from build123d import *

# Parameters (mm, degrees)
F2_R     = 6.35
F3_DEPTH = 6.732


with BuildPart() as f1:
    # F0 (on Front) → F1 (revolve)
    with BuildSketch(Plane.XZ):
        with BuildLine():
            Line((-7.5819, 0), (0, 0))
            Line((0, 0), (0, 6.731))
            Line((0, 6.731), (-7.062259, 6.731))
            ThreePointArc((-7.062259, 6.731), (-9.09525, 5.994764), (-10.1854, 4.1275))
            Line((-10.1854, 4.1275), (-8.2931, 4.1275))
            Line((-8.2931, 4.1275), (-8.2931, 2.6035))
            Line((-8.2931, 2.6035), (-10.1854, 2.6035))
            ThreePointArc((-10.1854, 2.6035), (-9.422853, 0.762547), (-7.5819, 0))
        make_face()
    revolve(axis=Axis((0, 0, 3.3655), (0, 0, 1)))

    # F2 (on face) → F3 (cut, through all)
    with BuildSketch(Plane.XY.offset(6.731)):
        Circle(F2_R)
    extrude(amount=-F3_DEPTH, mode=Mode.SUBTRACT)


solid = f1.part
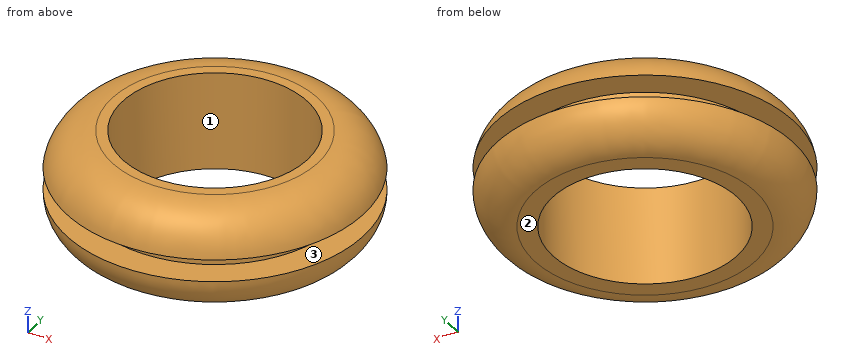
Read the model definition and answer for the solid it produces. Units are mm, in the model's axes. Face numbers are marked on the shaded views. Round coordinates to 2 decimals unless told otherwise and drop trailing zeros. Write each loop counter-clockwise with the first axis right and the second up, starting at its lowest first coordinate (ties: lowest second). Pieces come first, ordered by that corner, then holes. Notation, with made-up numbers: (-36.75, 19.25) - (-13.75, 19.25) arc R5 cw to (-13.75, 25.25) - close; hole circle Ø2 at (87, 26.25). An arc over 180 degrees is marked (long way). Use a Markdown table: item, result.
(1) Straight lines are drawn through the part: line 1 along Y through (x, z) = (0, 2.75); line 2 along Y through (x, z) = (0, 2.5); line 3 along Z through (x, y) = (-8.25, -4.5). For each, find the intervals that lie inside material, in ascending order. Write a range as [from, to].
Reported:
| item | result |
|---|---|
| line 1 | [-8.29, -6.35], [6.35, 8.29] |
| line 2 | [-10.18, -6.35], [6.35, 10.18] |
| line 3 | [0.74, 2.6], [4.13, 5.71] |
(2) The part is cut by section C-C (z = 5). Write down the section's boundary in (x, y).
Reported:
| item | result |
|---|---|
| outline | circle Ø19.78 at (0, 0); hole circle Ø12.7 at (0, 0) |
(3) The part is cut by section D-D (z = 1.5). Write down the section's boundary in (x, y).
Reported:
| item | result |
|---|---|
| outline | circle Ø19.88 at (0, 0); hole circle Ø12.7 at (0, 0) |
(4) The mould has two halves that part along Z. Classify the marked faces 1, 2 and 3: released by +Z, released by -Z, zero draft, split by the parting line, or undercut.
Reported:
| item | result |
|---|---|
| face 1 | zero draft |
| face 2 | released by -Z |
| face 3 | undercut |
(5) Each of these flat-tipped pins is pushed along its axis until it touches: pin 1 Ø1 at (y, z) = (3.5, 2) entering from -X; pin 2 Ø1.5 at (x, z) = (-3, 4) entering from +Y; pin 3 Ø2 at (y, z) = (-5, 2) entering from -X. Where does it stop, or does it pass through?
Reported:
| item | result |
|---|---|
| pin 1 | x = -9.69 |
| pin 2 | y = 9.93 |
| pin 3 | x = -9.33 |
